Model file for the job. Use its own axes, mm. Give positions to 0.01 mm unless a question says otherwise; leave off trailing zeros. Loops run counter-clockwise (first coordinate to the right, second up) from the corner with the lowest first, then second, coordinate; pieces in that order, holes last. Notation, with made-up numbers: M 19,11.5 L 35,11.5 A28 ccw 35,35.5 Z; hole C 2.5,-17.5 d2. An arc over 180 degrees is marked long. Answer in a Markdown table with one row per item.
Autodesk Inventor part; units mm, degrees
ref_plane "YZ Plane" through (0, 0, 0) normal (1, 0, 0) x (0, 1, 0)
ref_plane "XZ Plane" through (0, 0, 0) normal (0, 1, 0) x (-1, 0, 0)
ref_plane "XY Plane" through (0, 0, 0) normal (0, 0, 1) x (1, 0, 0)
sketch "Sketch1" plane through (0, 0, 0) normal (0, 0, 1) x (1, 0, 0)
  line L0 (-30.5, -25) -> (30.5, -25)
  line L1 (42.5, -13) -> (42.5, 13)
  line L2 (30.5, 25) -> (-30.5, 25)
  line L3 (-42.5, 13) -> (-42.5, -13)
  line L4 (-42.5, -25) -> (42.5, 25) construction
  line L5 (42.5, -25) -> (-42.5, 25) construction
  arc A0 (-30.5, 25) -> (-42.5, 13) centre (-30.5, 13) ccw
  arc A1 (-42.5, -13) -> (-30.5, -25) centre (-30.5, -13) ccw
  arc A2 (30.5, -25) -> (42.5, -13) centre (30.5, -13) ccw
  arc A3 (42.5, 13) -> (30.5, 25) centre (30.5, 13) ccw
  line L6 (-19.05, -19.05) -> (19.05, -19.05)
  line L7 (19.05, -19.05) -> (19.05, 19.05)
  line L8 (19.05, 19.05) -> (-19.05, 19.05)
  line L9 (-19.05, 19.05) -> (-19.05, -19.05)
  line L10 (-19.05, -19.05) -> (19.05, 19.05) construction
  line L11 (19.05, -19.05) -> (-19.05, 19.05) construction
  circle A4 centre (0, 0) radius 12.5
  line L12 (-19.05, 19.05) -> (-16.95, 19.05)
  line L13 (-16.95, 19.05) -> (-16.95, 16.95)
  circle A5 centre (-16.95, 16.95) radius 2.25
  line L14 (19.05, 19.05) -> (16.95, 19.05)
  line L15 (16.95, 19.05) -> (16.95, 16.95)
  line L16 (-19.05, -19.05) -> (-16.95, -19.05)
  line L17 (-16.95, -19.05) -> (-16.95, -16.95)
  line L18 (19.05, -19.05) -> (16.95, -19.05)
  line L19 (16.95, -19.05) -> (16.95, -16.95)
  circle A6 centre (16.95, 16.95) radius 2.25
  circle A7 centre (-16.95, -16.95) radius 2.25
  circle A8 centre (16.95, -16.95) radius 2.25
  line L20 (0, 0) -> (30.625, 0)
  line L21 (0, 0) -> (-30.625, 0)
  circle A9 centre (-30.625, 0) radius 3.2
  circle A10 centre (30.625, 0) radius 3.2
  circle A11 centre (0, 19.05) radius 2.85
  dimension "d0" = 85
  dimension "d1" = 50
  dimension "d2" = 12
  dimension "d3" = 38.1
  dimension "d4" = 38.1
  dimension "d5" = 25
  dimension "d6" = 2.1
  dimension "d7" = 2.1
  dimension "d8" = 4.5
  dimension "d9" = 2.1
  dimension "d10" = 2.1
  dimension "d11" = 2.1
  dimension "d12" = 2.1
  dimension "d13" = 2.1
  dimension "d14" = 2.1
  dimension "d15" = 4.5
  dimension "d16" = 4.5
  dimension "d17" = 4.5
  dimension "d18" = 30.625
  dimension "d19" = 30.625
  dimension "d20" = 6.4
  dimension "d21" = 6.4
  dimension "d22" = 5.7
extrude "Extrusion1" add sketch "Sketch1" against normal blind 6 contours A1 L3 A0 L2 A3 L1 A2 L0 | L9 A7 L6 | A9 | A10 | A7 L9 L6 | L6 A7 | A7 L9 | A7 L9 L21 A4 L20 L7 A8 L6 | A8 L7 L6 | L6 A8 | L9 A5 L8 A11 A6 L7 L20 A4 L21 | A8 L7 | A8 L7 L6 | A5 L9 | L9 A5 L8 | L21 L20 A4 | A4 L20 L21 | L9 L8 A5 | A6 L8 L7 | L7 A6 | A5 L8 | A6 L8 L7 | A6 L8 | A11 L8 | L8 A11
hole "Hole1" at (-30.625, 0, 0) at (30.625, 0, 0) direction (0, 0, -1) diameter 3.4 end through all
hole "Hole2" at (0, 19.05, 0) direction (0, 0, -1) diameter 2.459 end through all
hole "Hole3" at (-16.95, 16.95, 0) at (16.95, 16.95, 0) at (16.95, -16.95, 0) at (-16.95, -16.95, 0) direction (0, 0, -1) diameter 1.567 end through all
hole "Hole4" at (0, 0, 0) direction (0, 0, -1) diameter 25 end through all
sketch "Sketch2" plane through (0, 0, -6) normal (0, 0, -1) x (-1, 0, 0)
  line L0 (42.5, 25) -> (14.5, 25)
  line L1 (14.5, 25) -> (14.5, 1)
  line L2 (42.5, 25) -> (42.5, 16.73)
  line L3 (42.5, 16.73) -> (28.7, 16.73)
  line L4 (-42.5, -25) -> (-42.5, -16.73)
  line L5 (-42.5, -16.73) -> (-28.7, -16.73)
  line L6 (-42.5, -25) -> (-14.5, -25)
  line L7 (30.5, -25) -> (-30.5, -25)
  line L8 (-14.5, -25) -> (-14.5, -1)
  line L9 (-42.5, 25) -> (-12.5, 25)
  line L10 (-12.5, 25) -> (-12.5, 13)
  line L11 (42.5, -25) -> (12.5, -25)
  line L12 (12.5, -25) -> (12.5, -13)
  line L13 (-42.5, 25) -> (-42.5, 8)
  line L14 (-42.5, 8) -> (-33.11, 8)
  line L15 (42.5, -25) -> (42.5, -8)
  line L16 (42.5, -8) -> (33.11, -8)
  point P0 (0, 0)
  dimension "d53" = 28
  dimension "d54" = 24
  dimension "d55" = 8.27
  dimension "d56" = 13.8
  dimension "d57" = 8.27
  dimension "d58" = 13.8
  dimension "d59" = 28
  dimension "d60" = 24
  dimension "d61" = 30
  dimension "d62" = 12
  dimension "d63" = 30
  dimension "d64" = 12
  dimension "d65" = 17
  dimension "d66" = 9.39
  dimension "d67" = 17
  dimension "d68" = 9.39
hole "Hole5" at (33.11, 8, -6) at (12.5, 13, -6) at (-28.7, 16.73, -6) at (-14.5, 1, -6) at (-33.11, -8, -6) at (-12.5, -13, -6) at (14.5, -1, -6) at (28.7, -16.73, -6) direction (0, 0, 1) diameter 1.567 end through all
properties part number "new-adapter-plate"
Q1. Saw through at C-C (z = -4). Give the number of separate pieces and of enclosed holes in the cut face, and give its area (3 significant figures).
Reported:
| item | result |
|---|---|
| separate pieces | 1 |
| enclosed holes | 16 |
| area | 3,590 mm² |
Q2. Saw through at A-A (x = 0). Give the cut face in (y, z).
Reported:
| item | result |
|---|---|
| outline | M -25,-6 L -12.5,-6 L -12.5,0 L -25,0 Z; M 12.5,-6 L 17.82,-6 L 17.82,0 L 12.5,0 Z; M 20.28,-6 L 25,-6 L 25,0 L 20.28,0 Z |
Q3. Probe probe 1 along Y at (x, z) = (0, -3.2); probe 2 along X at (y, z) = (0, -3.75) (3 decimals); probe 3 along Y at (x, z) = (-16.95, -1.75). List the from-to ranges inside material, lowest first.
Reported:
| item | result |
|---|---|
| probe 1 | -25 to -12.5, 12.5 to 17.82, 20.28 to 25 |
| probe 2 | -42.5 to -32.325, -28.925 to -12.5, 12.5 to 28.925, 32.325 to 42.5 |
| probe 3 | -25 to -17.73, -16.17 to 16.17, 17.73 to 25 |
Q4. Mould opens along X. For faces 1 (the face through (0, 25, -3)), 2 (the face through (16.916, 17.733, -3.042)), 3 (the face through (-42.5, 0, -3)), 4 (the face through (-17.48, 17.527, -3.042)) say: released by +X, released by -X, zero draft, split by the parting line, or undercut.
Reported:
| item | result |
|---|---|
| face 1 | zero draft |
| face 2 | undercut |
| face 3 | released by -X |
| face 4 | undercut |
Q5. Saw through at B-B (x = 10). Give the cut face in (y, z), and give its area (3 significant figures).
Reported:
| item | result |
|---|---|
| outline | M -25,-6 L -7.5,-6 L -7.5,0 L -25,0 Z; M 7.5,-6 L 25,-6 L 25,0 L 7.5,0 Z |
| area | 210 mm² |
